Autodesk Inventor part; units mm, degrees
ref_plane "YZ Plane" through (0, 0, 0) normal (1, 0, 0) x (0, 1, 0)
ref_plane "XZ Plane" through (0, 0, 0) normal (0, 1, 0) x (-1, 0, 0)
ref_plane "XY Plane" through (0, 0, 0) normal (0, 0, 1) x (1, 0, 0)
sketch "Skizze1" plane through (0, 0, 0) normal (0, 0, 1) x (1, 0, 0)
  line L0 (0, 0) -> (53, 0)
  line L1 (53, 0) -> (53, 30)
  line L2 (53, 30) -> (0, 30)
  line L3 (0, 30) -> (0, 0)
  dimension "d0" = 30
  dimension "d1" = 53
extrude "Extrusion1" add sketch "Skizze1" along normal blind 2
sketch "Skizze2" plane through (0, 0, 2) normal (0, 0, 1) x (1, 0, 0)
  line L0 (0, 0) -> (53, 0)
  line L1 (53, 0) -> (53, 30)
  line L2 (53, 30) -> (0, 30)
  line L3 (0, 30) -> (0, 0)
  line L4 (2.5, 2.5) -> (50.5, 2.5)
  line L5 (50.5, 2.5) -> (50.5, 27.5)
  line L6 (50.5, 27.5) -> (2.5, 27.5)
  line L7 (2.5, 27.5) -> (2.5, 2.5)
  dimension "d4" = 25
  dimension "d5" = 48
  dimension "d6" = 2.5
  dimension "d7" = 2.5
  dimension "d8" = 2.5
  dimension "d9" = 2.5
extrude "Extrusion2" add sketch "Skizze2" along normal blind 16
sketch "Skizze8" plane through (0, 0, 18) normal (0, 0, 1) x (1, 0, 0)
  line L0 (50.5, 27.5) -> (50.5, 2.5)
  line L1 (53, 0) -> (53, 30)
  line L2 (50.5, 8.5) -> (53, 8.5)
  line L3 (53, 8.5) -> (53, 21.5)
  line L4 (53, 21.5) -> (50.5, 21.5)
  line L5 (50.5, 21.5) -> (50.5, 8.5)
  line L6 (0, 0) -> (53, 0)
  line L7 (53, 30) -> (0, 30)
  dimension "d49" = 13
  dimension "d50" = 8.5
  dimension "d51" = 8.5
extrude "Extrusion8" cut sketch "Skizze8" against normal blind 11
hole "Bohrung2" at (17.5, 15, 0) direction (0, 0, 1) diameter 3 end through all countersink diameter 4 countersink angle 90
sketch "Skizze9" plane through (0, 0, 18) normal (0, 0, 1) x (1, 0, 0)
  line L0 (2.5, 27.5) -> (2.5, 2.5)
  line L1 (0, 12.25) -> (2.5, 12.25)
  line L2 (2.5, 12.25) -> (2.5, 17.75)
  line L3 (2.5, 17.75) -> (0, 17.75)
  line L4 (0, 17.75) -> (0, 12.25)
  line L5 (0, 0) -> (53, 0)
  line L6 (53, 30) -> (0, 30)
  dimension "d63" = 5.5
  dimension "d64" = 12.25
  dimension "d65" = 12.25
extrude "Extrusion9" add sketch "Skizze9" along normal blind 1
fillet "Rundung2" radius 1 4 edges at (1.25, 12.25, 19) (1.25, 17.75, 19) (51.75, 21.5, 7) (51.75, 8.5, 7)
properties part number "V2_oberteil"
Model file for the job. Use its own axes, mm. A direction names the side the tool comes from. Give positions to 0.01 mm unless a question says otherwise; leave off trailing zeros. Loops run counter-clockwise (first coordinate to the right, second up) from the corner with the lowest first, then second, coordinate; pieces in that order, holes last. Notation, with made-up numbers: (48.5, 39) - (69.5, 39) arc R5 cw to (69.5, 44) - close; hole circle Ø3 at (89.25, 69.25). An arc over 180 degrees is marked (long way). One line per item, written item: value. Start each with the question number.
1. Probe L1, parallel to Y at x = 46.5, z = 15; L2, parallel to X at y = 15, z = 1.2; L3, parallel to Y at x = 17.5, z = 1.15. List the from-to ranges inside material, lowest first. Write a range as from..to.
2. Which spindle directions (+Z, -Z, +X, -X, +Y, -Y) get a long thin tool onto all of the face, cutting with end or side? Do faces 5 (the flat face through (24, 28, 18)), 6 (the flat face through (26, 2.5, 10)), 7 (the flat face through (52, 8.5, 13)). Say none if no direction does.
3. Slice it at B-B (x = 17.5). List the corners of the cut face in (y, z).
4. Slice it at C-C (z = 16.5). List the corners of the cut face in (x, y).
5. Slice it at D-D (x = 5.5). List the corners of the cut face in (y, z).
6. Pull direction X, two halves, no side cores. Call faces 1 (the flat face through (53, 15, 5)), 2 (the flat face through (50.5, 15, 6)), 3 (the flat face through (24, 2, 18)), 4 (the flat face through (27, 27.5, 10)): pulls with the +X half, pulls with the -X half, needs draft (parallel to the pull), parting line crosses it, or undercut.
7. Slice it at A-A (y = 15). List the corners of the cut face in (x, z).
8. Pin check, flat tips, straight feed: pin 1 (5 mm diameter, centred on x = 18, y = 22.5, fed in from +Z); pin 2 (10 mm diameter, centred on x = 15.5, y = 3, fed in from +Z); pin 3 (2.5 mm diameter, centred on x = 17.5, y = 15, fed in from -Z); pin 4 (3 mm diameter, centred on x = 52, y = 15, fed in from +Z). Stop position of each tip, or through.
Solution:
1. L1: y = 0..2.5, 27.5..30
1. L2: x = 0..16, 19..53
1. L3: y = 0..13.5, 16.5..30
2. face 5: +Z, +X, -X, +Y
2. face 6: +Z
2. face 7: +Z, +X
3. outline: (0, 0) - (13, 0) - (13.5, 0.5) - (13.5, 2) - (2.5, 2) - (2.5, 18) - (0, 18) - close; (16.5, 0.5) - (17, 0) - (30, 0) - (30, 18) - (27.5, 18) - (27.5, 2) - (16.5, 2) - close
4. outline: (0, 0) - (53, 0) - (53, 8.5) - (50.5, 8.5) - (50.5, 2.5) - (2.5, 2.5) - (2.5, 27.5) - (50.5, 27.5) - (50.5, 21.5) - (53, 21.5) - (53, 30) - (0, 30) - close
5. outline: (0, 0) - (30, 0) - (30, 18) - (27.5, 18) - (27.5, 2) - (2.5, 2) - (2.5, 18) - (0, 18) - close
6. face 1: pulls with the +X half
6. face 2: undercut
6. face 3: needs draft
6. face 4: undercut
7. outline: (0, 0) - (15.5, 0) - (16, 0.5) - (16, 2) - (2.5, 2) - (2.5, 19) - (0, 19) - close; (19, 0.5) - (19.5, 0) - (53, 0) - (53, 7) - (50.5, 7) - (50.5, 2) - (19, 2) - close
8. pin 1: stops at z = 2
8. pin 2: stops at z = 18
8. pin 3: passes through
8. pin 4: stops at z = 7
